Work out the finished part from the listing and answer in its coordinate system (mm). Face numbers are marked on the shaded views. A direction names the side the tool comes from. Coordinates: 2 decimals unless noted, no trailing zeros. Write each loop counter-clockwise with the first axis right and the second up, starting at its lowest first coordinate (ties: lowest second). Pieces come first, ordered by that corner, then holes. Notation, with made-up numbers: (62.5, 8) - (76.5, 8) arc R16 ccw to (76.5, 34) - close; hole circle Ø2 at (19.25, -22.5). An arc over 180 degrees is marked (long way). Answer as a JSON object with one key per item and string values. Group by question number.
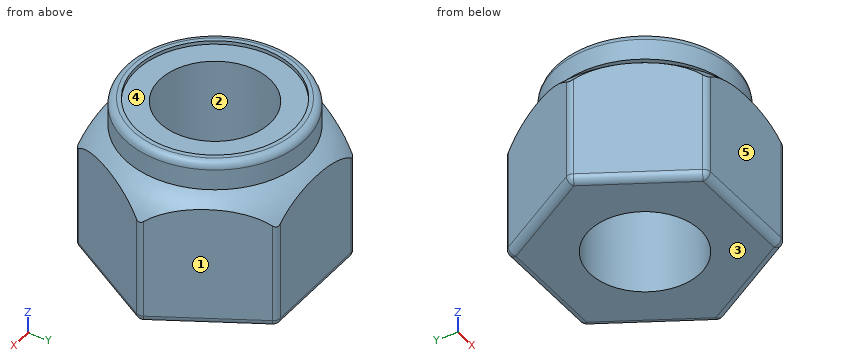
Autodesk Inventor part; units mm, degrees
ref_plane "YZ Plane" through (0, 0, 0) normal (1, 0, 0) x (0, 1, 0)
ref_plane "XZ Plane" through (0, 0, 0) normal (0, 1, 0) x (-1, 0, 0)
ref_plane "XY Plane" through (0, 0, 0) normal (0, 0, 1) x (1, 0, 0)
sketch "Sketch1" plane through (0, 0, 0) normal (0, 0, 1) x (1, 0, 0)
  line L0 (-4.1244, 7.1437) -> (4.1244, 7.1437)
  line L1 (4.1244, 7.1437) -> (8.2489, 0)
  line L2 (8.2489, 0) -> (4.1244, -7.1437)
  line L3 (4.1244, -7.1437) -> (-4.1244, -7.1437)
  line L4 (-4.1244, -7.1437) -> (-8.2489, 0)
  line L5 (-8.2489, 0) -> (-4.1244, 7.1437)
  point P0 (0, 0)
  point P1 (0, 0)
  dimension "d0" = 14.2875
extrude "Extrusion1" add sketch "Sketch1" along normal blind 9.525
sketch "Sketch3" plane through (0, 0, 9.525) normal (0, 0, 1) x (1, 0, 0)
  circle A0 centre (0, 0) radius 6.35
  dimension "d3" = 12.7
extrude "Extrusion2" add sketch "Sketch3" along normal blind 1.9844
sketch "Sketch8" plane through (0, 0, 11.5094) normal (0, 0, 1) x (1, 0, 0)
  circle A0 centre (0, 0) radius 6.35
  circle A1 centre (0, 0) radius 5.5563
  circle A2 centre (0, 0) radius 5.1594
  dimension "d14" = 11.1125
  dimension "d28" = 10.3187
extrude "Extrusion3" cut sketch "Sketch8" against normal blind 0.254 contours A1 | A2
sketch "Sketch9" plane through (0, 0, 0) normal (0, 0, -1) x (-1, 0, 0)
  point P0 (0, 0)
hole "Hole2" at (0, 0, 0) direction (0, 0, 1) diameter 7.7978 end through all
sketch "Sketch10" plane through (0, 0, 0) normal (0, 1, 0) x (-1, 0, 0)
  line L0 (-8.2489, 9.525) -> (-4.1244, 9.525)
  line L1 (-4.1244, 0) -> (-4.1244, 9.525)
  line L2 (-8.2489, 0) -> (-4.1244, 0)
  line L3 (-8.2489, 0) -> (-8.2489, 9.525)
  line L4 (0, 0) -> (0, 6.9243)
  arc A0 (-4.572, 9.525) -> (-8.2489, 7.3406) centre (-4.572, 5.3382) ccw
  line L5 (-8.2489, 7.3406) -> (-8.2489, 9.525)
  line L6 (-4.572, 9.525) -> (-8.2489, 9.525)
  dimension "d24" = 4.572
revolve "Revolution2" cut sketch "Sketch10" angle 360 about axis through (0, 0, 0) along (0, 0, 1) contours L0 A0 L3
fillet "Fillet1" radius 0.508 12 edges at (-4.1244, -7.1437, 3.6703) (4.1244, -7.1437, 3.6703) (8.2489, 0, 3.6703) (4.1244, 7.1437, 3.6703) (-8.2489, 0, 3.6703) (-4.1244, 7.1437, 3.6703) (0, 7.1437, 0) (6.1867, 3.5719, 0) (6.1867, -3.5719, 0) (0, -7.1437, 0) (-6.1867, -3.5719, 0) (-6.1867, 3.5719, 0)
fillet "Fillet2" radius 0.508 1 edges at (-6.35, 0, 11.5094)
properties part number "10-32 regular lock nut" material "Steel"
Q1. Flat-ended cylindrical pins translate along their axes: pin 1 Ø2 at (x, y) = (1, -2) entering from +Z; pin 2 Ø6 at (y, z) = (-5, 6) entering from -X; pin 3 Ø1.5 at (x, y) = (-4, 1.5) entering from -Z. Find the tip coordinate at first contact, or state that the pin passes through.
Q2. Section C-C on z = 10 is taken. Determine the outline of the cut face in (x, y), plus the area to 3 significant figures.
Q3. Consider L1, parallel to Y at x = 0, z = 4.5; L2, parallel to Y at x = 0.75, z = 4.25; L3, parallel to X at y = 0, z = 4.5. Determine where each line is inside the solid, lowest interval first. Write a range as from..to.
Q4. Section A-A on z = 6 is taken. Determine the outline of the cut face in (x, y).
Q5. A tool of negligible diameter and unlimited length cuts with its end or side. For the marked faces 4 and 5, from which of +Z, -Z, +X, -X, +Y, -Y can it reach the whole face along a straight path? Write none if from no direction.
Q6. Section B-B on x = 0 is taken. Determine the outline of the cut face in (y, z) (3 decimals).
Q7. For a pull along X with two mould halves and no side action, classify the marked faces 1, 2 and 3 as +X half, -X half, draft (parallel to the pull), parting line (faces both ways), or undercut.
Numbers:
{
 "1": {"pin 1": "passes through", "pin 2": "stops at x = -7.09", "pin 3": "stops at z = 0"},
 "2": {"outline": "circle Ø12.7 at (0, 0); hole circle Ø7.8 at (0, 0)", "area": "78.9 mm²"},
 "3": {"L1": "y = -7.14..-3.9, 3.9..7.14", "L2": "y = -7.14..-3.83, 3.83..7.14", "L3": "x = -8.17..-3.9, 3.9..8.17"},
 "4": {"outline": "(-8.1, -0.25) - (-4.27, -6.89) arc R0.51 ccw to (-3.83, -7.14) - (3.83, -7.14) arc R0.51 ccw to (4.27, -6.89) - (8.1, -0.25) arc R0.51 ccw to (8.1, 0.25) - (4.27, 6.89) arc R0.51 ccw to (3.83, 7.14) - (-3.83, 7.14) arc R0.51 ccw to (-4.27, 6.89) - (-8.1, 0.25) arc R0.51 ccw to start; hole circle Ø7.8 at (0, 0)"},
 "5": {"face 4": "+Z", "face 5": "+Z, -Z, +X, -X, -Y"},
 "6": {"outline": "(-7.144, 0.508) arc R0.508 ccw to (-6.636, 0) - (-3.899, 0) - (-3.899, 11.255) - (-5.556, 11.255) - (-5.556, 11.509) - (-5.842, 11.509) arc R0.508 ccw to (-6.35, 11.001) - (-6.35, 9.525) - (-4.572, 9.525) arc R4.187 ccw to (-7.144, 8.642) - close; (3.899, 0) - (6.636, 0) arc R0.508 ccw to (7.144, 0.508) - (7.144, 8.642) arc R4.187 ccw to (4.572, 9.525) - (6.35, 9.525) - (6.35, 11.001) arc R0.508 ccw to (5.842, 11.509) - (5.556, 11.509) - (5.556, 11.255) - (3.899, 11.255) - close"},
 "7": {"face 1": "+X half", "face 2": "undercut", "face 3": "draft"}
}
